Source: CAD feature listing. Evaluate the final solid. Frame: model axes, mm. Face numbers are marked on the shaded views. Round coordinates to 2 decimals unless told otherwise and drop trailing zeros. Write each loop counter-clockwise with the first axis right and the second up, starting at its lowest first coordinate (ties: lowest second). Pieces come first, ordered by that corner, then holes. Notation, with made-up numbers: (38.5, 48.25) - (96.5, 48.25) arc R3 cw to (96.5, 53.25) - close; hole circle Ø11 at (-19, -26). An arc over 180 degrees is marked (long way). Write item = value, one per line. Start each with the question number.
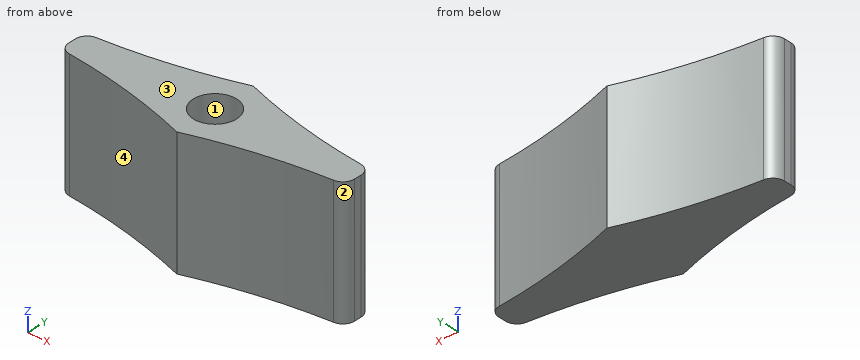
```python
from build123d import *

# Parameters (mm, degrees)
F0_R     = 3.75
F0_R_2   = 3
F1_DEPTH = 22
F2_R     = 3
F3_DEPTH = 20
F2_R_2   = 3.75
F4_DEPTH = 15


with BuildPart() as f1:
    # F0 (on Top) → F1 (new body)
    with BuildSketch(Plane.XY):
        with BuildLine():
            ThreePointArc((23.177466, -2.64573), (24.475624, -2.003632), (25, -0.653619))
            Line((25, -0.653619), (25, 0.653619))
            ThreePointArc((25, 0.653619), (24.475624, 2.003632), (23.177466, 2.64573))
            ThreePointArc((23.177466, 2.64573), (11.445847, 4.390631), (0, 7.5))
            ThreePointArc((0, 7.5), (-11.445847, 4.390631), (-23.177466, 2.64573))
            ThreePointArc((-23.177466, 2.64573), (-24.475624, 2.003632), (-25, 0.653619))
            Line((-25, 0.653619), (-25, -0.653619))
            ThreePointArc((-25, -0.653619), (-24.475624, -2.003632), (-23.177466, -2.64573))
            ThreePointArc((-23.177466, -2.64573), (-11.445847, -4.390631), (0, -7.5))
            ThreePointArc((0, -7.5), (11.445847, -4.390631), (23.177466, -2.64573))
        make_face()
        Circle(F0_R, mode=Mode.SUBTRACT)
        Circle(F0_R)
        Circle(F0_R_2, mode=Mode.SUBTRACT)
        Circle(F0_R_2)
    extrude(amount=F1_DEPTH)

    # F2 (on face) → F3 (cut)
    with BuildSketch(Plane.XY.offset(22)):
        Circle(F2_R)
    extrude(amount=-F3_DEPTH, mode=Mode.SUBTRACT)

    # F2 (on face) → F4 (cut)
    with BuildSketch(Plane.XY.offset(22)):
        Circle(F2_R_2)
        Circle(F2_R, mode=Mode.SUBTRACT)
    extrude(amount=-F4_DEPTH, mode=Mode.SUBTRACT)


solid = f1.part
```
(1) Section B-B (y = 0). Return the cut outline in (x, z), plus the area to 4 significant figures.
(2) Pull-direction query (X, two-part tool) for the marked faces 1, 2, 3 and 4; classes: +X half, -X half, draft (parallel to the pull), parting line (faces both ways), or undercut.
(3) Section D-D (y = 6). Return the cut outline in (x, z), plus the area to 3 significant figures.
(4) Section A-A (z = 14). Return the cut outline in (x, y).
(5) Contact query for flat-ended pins moving along their axis: P1, Ø1.8, axis at x = -0.5, y = 0.5, coming from the +Z side; P2, Ø4, axis at x = -13.5, z = 4.5, coming from the -Y side; P3, Ø6, axis at x = -0.5, y = 0.5, coming from the +Z side. Output: stop coordinate, or through.
(6) Section C-C (x = -0.5). Return the cut outline in (y, z), plus the area to 3 significant figures.
(7) Ray query, L1, parallel to Y at x = 0, z = 14.25; L2, parallel to Y at x = 0, z = 5.25; L3, parallel to X at y = 1.75, z = 16. Return the intervals inside material, ascending. Write a range as from..to.
Solution:
q1.outline = (-25, 0) - (25, 0) - (25, 22) - (3.75, 22) - (3.75, 7) - (3, 7) - (3, 2) - (-3, 2) - (-3, 7) - (-3.75, 7) - (-3.75, 22) - (-25, 22) - close
q1.area = 957.5 mm^2
q2.face_1 = undercut
q2.face_2 = +X half
q2.face_3 = draft
q2.face_4 = -X half
q3.outline = (-4.87, 0) - (4.87, 0) - (4.87, 22) - (-4.87, 22) - close
q3.area = 214 mm^2
q4.outline = (-25, -0.65) arc R2 ccw to (-23.18, -2.65) arc R100.91 cw to (0, -7.5) arc R100.91 cw to (23.18, -2.65) arc R2 ccw to (25, -0.65) - (25, 0.65) arc R2 ccw to (23.18, 2.65) arc R100.91 cw to (0, 7.5) arc R100.91 cw to (-23.18, 2.65) arc R2 ccw to (-25, 0.65) - close; hole circle Ø7.5 at (0, 0)
q5.P1 = 2
q5.P2 = -4.38
q5.P3 = 7
q6.outline = (-7.33, 0) - (7.33, 0) - (7.33, 22) - (3.72, 22) - (3.72, 7) - (2.96, 7) - (2.96, 2) - (-2.96, 2) - (-2.96, 7) - (-3.72, 7) - (-3.72, 22) - (-7.33, 22) - close
q6.area = 182 mm^2
q7.L1 = -7.5..-3.75, 3.75..7.5
q7.L2 = -7.5..-3, 3..7.5
q7.L3 = -24.67..-3.32, 3.32..24.67
